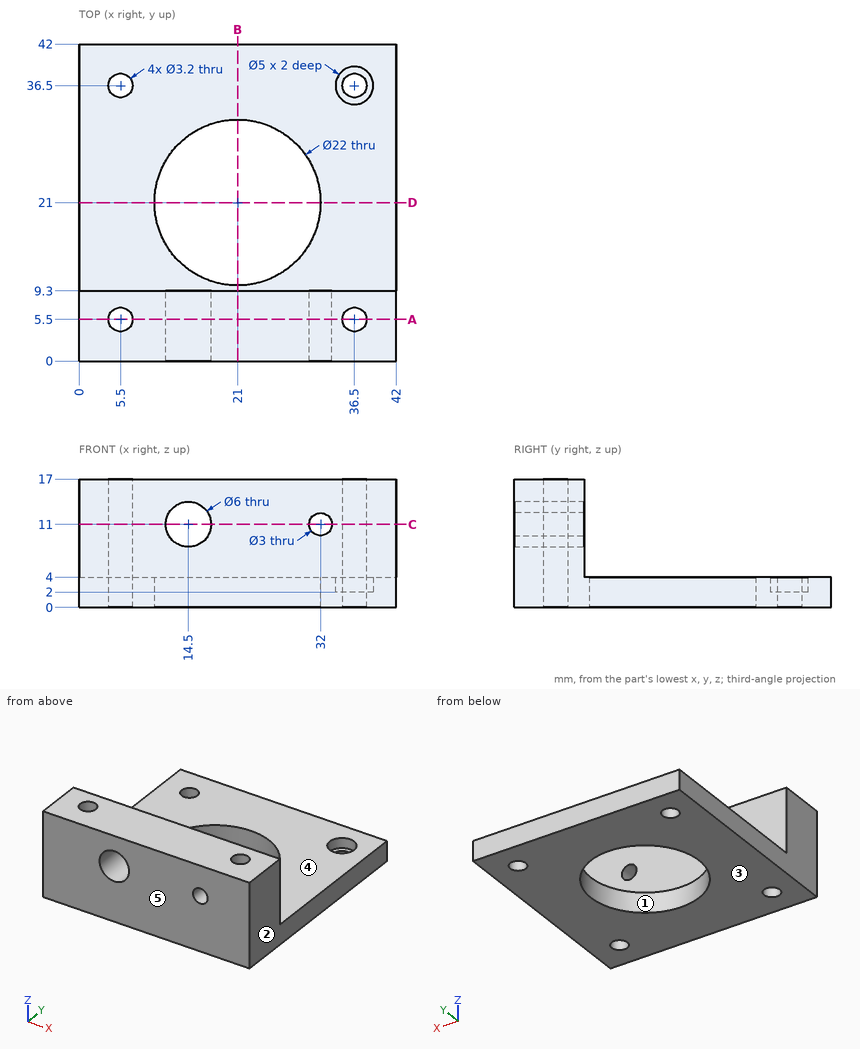
Study the drawing (mm; zero at the part's minimum x, y, z) and answer. A direction names the side the tool comes from. Round coordinates to 2 decimals unless told otherwise and drop trailing zeros. Write each loop counter-clockwise with the first axis right and the second up, starting at its lowest first coordinate (ties: lowest second). Pieces come first, ordered by that corner, then holes. Notation, with made-up numbers: (0, 70) -> (34, 70) arc R19 cw to (34, 77) -> close; hole circle Ø6 at (16, 8.25). An arc over 180 degrees is marked (long way). Answer as CSV lines item,"result". Start each with the question number.
(1) The part is cut by section B-B, the plane x = 21. Give the vertices of the cut face in (y, z).
(2) Each of these flat-tipped pins is pushed along its axis until it touches: pin 1 (16.5 mm diameter, centred on x = 14, y = 23, fed in from +Z); pin 2 (2 mm diameter, centred on x = 32, z = 5.5, fed in from +Y). Where does it stop, or does it pass through?
(3) The mould has two halves that part along X. Classify the marked faces 1, 2 and 3: +X half, -X half, draft (parallel to the pull), parting line (faces both ways), or undercut.
(4) Find the intervals of material crossed by probe 1 along Y at (x, z) = (36.5, 1.25); probe 2 along Y at (x, z) = (36.5, 6.5), in increasing order.
(5) The part is cut by section C-C, the plane z = 11. Give the vertices of the cut face in (x, y), then the cut area to 3 significant figures.
(6) The part is cut by section D-D, the plane y = 21. Give the vertices of the cut face in (x, z).
(7) The part is cut by section A-A, the plane y = 5.5. Give the vertices of the cut face in (x, z).
(8) A tool of negligible diameter and unlimited length cuts with its end or side. For the marked faces 4 and 5, from which of +Z, -Z, +X, -X, +Y, -Y can it reach the whole face along a straight path? Write none if from no direction.
Output values:
1,outline,"(0, 0) -> (10, 0) -> (10, 4) -> (9.3, 4) -> (9.3, 17) -> (0, 17) -> close; (32, 0) -> (42, 0) -> (42, 4) -> (32, 4) -> close"
2,pin 1,"stops at z = 4"
2,pin 2,"stops at y = 9.3"
3,face 1,"undercut"
3,face 2,"+X half"
3,face 3,"draft"
4,probe 1,"y = 0 to 3.9, 7.1 to 34.9, 38.1 to 42"
4,probe 2,"y = 0 to 3.9, 7.1 to 9.3"
5,outline,"(0, 0) -> (11.5, 0) -> (11.5, 9.3) -> (0, 9.3) -> close; (17.5, 0) -> (30.5, 0) -> (30.5, 9.3) -> (17.5, 9.3) -> close; (33.5, 0) -> (42, 0) -> (42, 9.3) -> (33.5, 9.3) -> close; hole circle Ø3.2 at (5.5, 5.5); hole circle Ø3.2 at (36.5, 5.5)"
5,area,"291 mm²"
6,outline,"(0, 0) -> (10, 0) -> (10, 4) -> (0, 4) -> close; (32, 0) -> (42, 0) -> (42, 4) -> (32, 4) -> close"
7,outline,"(0, 0) -> (3.9, 0) -> (3.9, 17) -> (0, 17) -> close; (7.1, 0) -> (34.9, 0) -> (34.9, 17) -> (7.1, 17) -> close; (38.1, 0) -> (42, 0) -> (42, 17) -> (38.1, 17) -> close; hole circle Ø6 at (14.5, 11); hole circle Ø3 at (32, 11)"
8,face 4,"+Z, +X, -X, +Y"
8,face 5,"+Z, -Z, +X, -X, -Y"
